Model file for the job. Use its own axes, mm. Face numbers are marked on the shaded views. A direction names the side the tool comes from. Give positions to 0.01 mm unless a question says otherwise; leave off trailing zeros. Order: outer loops, then holes, each group sorted by start corner. A loop starts at its lowest first (then second) coordinate and runs counter-clockwise, first axis right, second up. Notation, with made-up numbers: (-32, 73) - (-3, 73) arc R15 ccw to (-3, 100) - close; hole circle Ø3 at (23.25, 16.5). An arc over 180 degrees is marked (long way). Use CSV: the item, a comma, the result in double quotes. Start each with the question number.
(1) Band-saw the part on B-B, the plane z = -10.5. Give the cut face in (x, y), then the cut area to 3 significant figures.
(2) Pull direction Z, two halves, no side cores. Call the marked faces 3, 4, 5 and 6: +Z half, -Z half, draft (parallel to the pull), parting line (faces both ways), or undercut.
(3) Band-saw the part on D-D, the plane x = 0. Give the cut face in (y, z).
(4) Drop flat-ended pins along their axis: pin 1 Ø0.8 at (x, z) = (-4, 13.5) entering from +Y; pin 2 Ø0.8 at (y, z) = (27, 13.5) entering from +X; pin 3 Ø0.5 at (y, z) = (38.5, 13.5) entering from +X; pin 4 Ø4 at (x, z) = (10.5, -0.5) entering from -Y. Give the stop position or say it passes through.
(5) Tool access for the marked faces 1 and 2: list every direction of +Z, -Z, +X, -X, +Y, -Y with a clear straight run to the whole face (end or side of a thin tool).
(6) Band-saw the part on A-A, the plane y = 27.5. Give the cut face in (x, z).
(7) Probe L1, parallel to Z at x = 2.5, y = 36; L2, parallel to X at y = 17.5, z = 6.5; L3, parallel to Y at x = 10, z = 2.5. List the from-to ranges inside material, lowest first.
(8) Band-saw the part on C-C, the plane x = 4. Give the cut face in (y, z), then the cut area to 3 significant figures.
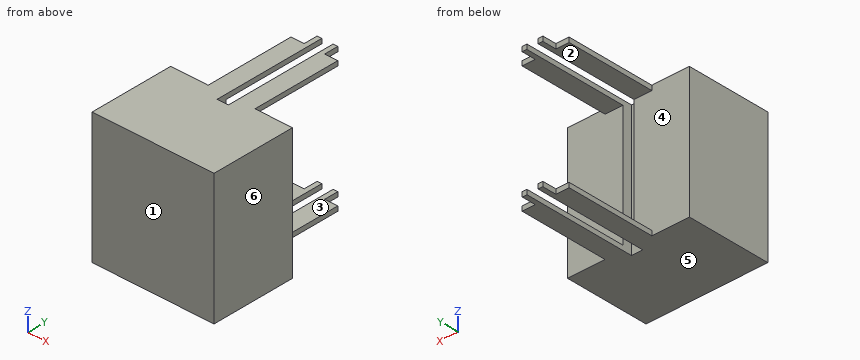
Autodesk Inventor part; units mm, degrees
ref_plane "YZ Plane" through (0, 0, 0) normal (1, 0, 0) x (0, 1, 0)
ref_plane "XZ Plane" through (0, 0, 0) normal (0, 1, 0) x (-1, 0, 0)
ref_plane "XY Plane" through (0, 0, 0) normal (0, 0, 1) x (1, 0, 0)
sketch "Sketch1" plane through (0, 0, 0) normal (0, 1, 0) x (-1, 0, 0)
  point P0 (0, 0)
sketch "Sketch2" plane through (0, 0, 0) normal (0, 1, 0) x (-1, 0, 0)
  line L0 (-13, 14) -> (13, 14)
  line L1 (13, 14) -> (13, -14)
  line L2 (13, -14) -> (-13, -14)
  line L3 (-13, -14) -> (-13, 14)
  line L4 (-13, 14) -> (13, -14) construction
  line L5 (13, 14) -> (-13, -14) construction
  point P0 (0, 0)
  dimension "d0" = 26
  dimension "d1" = 28
extrude "Extrusion1" add sketch "Sketch2" along normal blind 18
sketch "Sketch5" plane through (13, 0, 14) normal (1, 0, 0) x (0, 0, -1)
  point P0 (14, 0)
  point P1 (17, 39.5)
  point P2 (11, 39.5)
sketch "Sketch7" plane through (0, 18, 0) normal (0, 1, 0) x (1, 0, 0)
  point P0 (0, 0)
sketch "Sketch8" plane through (0, 18, 0) normal (0, 1, 0) x (1, 0, 0)
  line L0 (13, 14) -> (-13, 14)
  line L1 (13, 14) -> (5, 14)
  line L2 (-5, 14) -> (-4, 14)
  line L3 (-5, 14) -> (5, 14)
  line L4 (5, 14) -> (5, 13)
  line L5 (5, 13) -> (-5, 13)
  line L6 (-5, 13) -> (-5, 14)
  line L7 (-13, -14) -> (13, -14)
  line L8 (-5, -14) -> (5, -14)
  line L9 (5, -14) -> (5, -13)
  line L10 (5, -13) -> (-5, -13)
  line L11 (-5, -13) -> (-5, -14)
  point P0 (0, 0)
  dimension "d22" = 8
  dimension "d23" = 8
  dimension "d24" = 1
  dimension "d26" = 10
  dimension "d27" = 1
extrude "Extrusion5" add sketch "Sketch8" along normal blind 22
sketch "Sketch9" plane through (-13, 0, 14) normal (0, 0, 1) x (1, 0, 0)
  line L0 (8, 40) -> (18, 40)
  line L1 (10.7548, 39.8791) -> (11.7548, 39.8791) construction
  line L2 (11.7548, 15.8791) -> (14.1548, 15.8791)
  line L3 (14.1548, 15.8791) -> (14.1548, 40)
  line L4 (11.7548, 15.8791) -> (11.7548, 39.8791)
  line L5 (8, 40) -> (10.8, 40)
  line L6 (10.8, 40) -> (10.8, 37)
  line L7 (10.8, 37) -> (8, 37)
  line L8 (8, 37) -> (8, 40)
  line L9 (18, 40) -> (15.2, 40)
  line L10 (15.2, 40) -> (15.2, 37)
  line L11 (15.2, 37) -> (18, 37)
  line L12 (18, 37) -> (18, 40)
  point P0 (13, 0)
  dimension "d38" = 2.4
  dimension "d39" = 2.8
  dimension "d40" = 3
  dimension "d41" = 2.8
extrude "Extrusion6" cut sketch "Sketch9" along normal mid plane 100
sketch "Sketch10" plane through (-13, 0, 14) normal (0, 0, 1) x (1, 0, 0)
  line L0 (10.8, 40) -> (10.8, 37)
  line L1 (11.8, 40) -> (11.8, 16)
  line L2 (11.8, 16) -> (14.2, 16)
  line L3 (14.2, 16) -> (14.2, 40)
  line L4 (11.8, 40) -> (14.2, 40)
  line L5 (15.2, 40) -> (10.8, 40)
  point P0 (13, 0)
  dimension "d44" = 1
  dimension "d45" = 24
  dimension "d46" = 2.4
extrude "Extrusion7" cut sketch "Sketch10" along normal mid plane 100
properties part number "Suporte_motor"
Answer block:
1,outline,"(-13, 0) - (13, 0) - (13, 18) - (1.2, 18) - (1.2, 16) - (-1.2, 16) - (-1.2, 18) - (-13, 18) - close"
1,area,"463 mm2"
2,face 3,"undercut"
2,face 4,"undercut"
2,face 5,"-Z half"
2,face 6,"draft"
3,outline,"(0, -14) - (16, -14) - (16, 14) - (0, 14) - close"
4,pin 1,"stops at y = 37"
4,pin 2,"stops at x = 5"
4,pin 3,"stops at x = 2.2"
4,pin 4,"stops at y = 0"
5,face 1,"+Z, -Z, +X, -X, -Y"
5,face 2,"+X, -X, +Y"
6,outline,"(-5, -14) - (-1.2, -14) - (-1.2, -13) - (-5, -13) - close; (-5, 13) - (-1.2, 13) - (-1.2, 14) - (-5, 14) - close; (1.2, -14) - (5, -14) - (5, -13) - (1.2, -13) - close; (1.2, 13) - (5, 13) - (5, 14) - (1.2, 14) - close"
7,L1,"z = -14 to -13, 13 to 14"
7,L2,"x = -13 to -1.2, 1.2 to 13"
7,L3,"y = 0 to 18"
8,outline,"(0, -14) - (37, -14) - (37, -13) - (18, -13) - (18, 13) - (37, 13) - (37, 14) - (0, 14) - close"
8,area,"542 mm2"
